from build123d import *

# Parameters (mm, degrees)
BOSS_EXTRUDE1_DEPTH = 3
CUT_EXTRUDE1_DEPTH  = 10


with BuildPart() as part:
    # Sketch2 → Boss-Extrude1 (new body)
    with BuildSketch(Plane.XY):
        with BuildLine():
            Line((-53.128634422, -19.547588701), (-62.746809975, -19.547588701))
            Line((-62.746809975, -19.547588701), (-126.203620945, -19.547588701))
            Line((-126.203620945, -19.547588701), (-126.203620945, 48.452411299))
            ThreePointArc((-126.203620945, 48.452411299), (-118.881290474, 66.130080829), (-101.203620945, 73.452411299))
            Line((-101.203620945, 73.452411299), (-43.703620945, 73.452411299))
            ThreePointArc((-43.703620945, 73.452411299), (-26.025951415, 66.130080829), (-18.703620945, 48.452411299))
            Line((-18.703620945, 48.452411299), (-18.703620945, -51.547588701))
            ThreePointArc((-18.703620945, -51.547588701), (-26.025951415, -69.225258231), (-43.703620945, -76.547588701))
            Line((-43.703620945, -76.547588701), (-101.203620945, -76.547588701))
            ThreePointArc((-101.203620945, -76.547588701), (-118.881290474, -69.225258231), (-126.203620945, -51.547588701))
            Line((-126.203620945, -51.547588701), (-126.203620945, -31.547588701))
            Line((-126.203620945, -31.547588701), (-62.746809975, -31.547588701))
            Line((-62.746809975, -31.547588701), (-53.128634422, -31.547588701))
            ThreePointArc((-53.128634422, -31.547588701), (-47.128634422, -25.547588701), (-53.128634422, -19.547588701))
        make_face()
    extrude(amount=BOSS_EXTRUDE1_DEPTH)

    # Sketch3 → Cut-Extrude1 (cut)
    with BuildSketch(Plane.XY.offset(3)):
        with BuildLine():
            Line((-61.448620945, -37.476562772), (-61.448620945, -68.6318397))
            ThreePointArc((-61.448620945, -68.6318397), (-63.323620945, -70.5068397), (-65.198620945, -68.6318397))
            Line((-65.198620945, -68.6318397), (-65.198620945, -37.476562772))
            ThreePointArc((-65.198620945, -37.476562772), (-63.323620945, -35.601562772), (-61.448620945, -37.476562772))
        make_face()
        with BuildLine():
            Line((-83.458620945, -37.476562772), (-83.458620945, -68.6318397))
            ThreePointArc((-83.458620945, -68.6318397), (-81.583620945, -70.5068397), (-79.708620945, -68.6318397))
            Line((-79.708620945, -68.6318397), (-79.708620945, -37.476562772))
            ThreePointArc((-79.708620945, -37.476562772), (-81.583620945, -35.601562772), (-83.458620945, -37.476562772))
        make_face()
        with BuildLine():
            Line((-83.458620945, -13.61861463), (-83.458620945, 17.536662297))
            ThreePointArc((-83.458620945, 17.536662297), (-81.583620945, 19.411662297), (-79.708620945, 17.536662297))
            Line((-79.708620945, 17.536662297), (-79.708620945, -13.61861463))
            ThreePointArc((-79.708620945, -13.61861463), (-81.583620945, -15.49361463), (-83.458620945, -13.61861463))
        make_face()
        with BuildLine():
            Line((-61.448620945, -13.61861463), (-61.448620945, 17.536662297))
            ThreePointArc((-61.448620945, 17.536662297), (-63.323620945, 19.411662297), (-65.198620945, 17.536662297))
            Line((-65.198620945, 17.536662297), (-65.198620945, -13.61861463))
            ThreePointArc((-65.198620945, -13.61861463), (-63.323620945, -15.49361463), (-61.448620945, -13.61861463))
        make_face()
    extrude(amount=-CUT_EXTRUDE1_DEPTH, mode=Mode.SUBTRACT)


solid = part.part
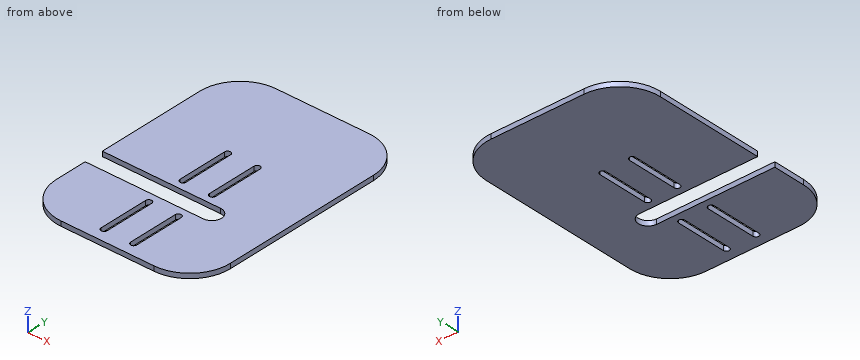
Read the model definition and answer for the solid it produces. Units are mm, in the model's axes. Give positions to 0.01 mm unless a question says otherwise; leave off trailing zeros. Write each loop counter-clockwise with the first axis right and the second up, starting at its lowest first coordinate (ties: lowest second). Pieces come first, ordered by that corner, then holes. Notation, with made-up numbers: (22, -34.75) - (61, -34.75) arc R17 ccw to (61, -16.75) - close; hole circle Ø10 at (16.5, 51). An arc over 180 degrees is marked (long way). Use CSV: the item, a comma, the result in double quotes. Start each with the question number.
(1) Find section D-D (x = -51). Give the vertices of the cut face in (y, z).
(2) Find section B-B (y = 14). Give the vertices of the cut face in (x, z), plus the area to 3 significant figures.
(3) Find section A-A (x = -68.5). Give the vertices of the cut face in (y, z), plus the area to 3 significant figures.
(4) Find section C-C (z = 1.15). Give the vertices of the cut face in (x, y) (3 decimals).
(5) Given P1, Ø1.5, axis at x = -71, y = 18, coming from the -Z side; P2, Ø1.5, axis at y = -60.5, z = 1.5, coming from the -X side, each flat-ended and moving along its own axis, determine where each tip first touches the part or whether it passes through.
(6) Consider line 1 along X through (y, z) = (8, 2.8); line 2 along Y through (x, z) = (-84.5, 1.55); line 3 along X through (y, z) = (-65.5, 0.3). Determine where each line is inside the solid, lowest interval first.
Findings below:
1,outline,"(-76.55, 0) - (-31.16, 0) - (-31.16, 3) - (-76.55, 3) - close; (-19.94, 0) - (73.45, 0) - (73.45, 3) - (-19.94, 3) - close"
2,outline,"(-126.2, 0) - (-83.46, 0) - (-83.46, 3) - (-126.2, 3) - close; (-79.71, 0) - (-65.2, 0) - (-65.2, 3) - (-79.71, 3) - close; (-61.45, 0) - (-18.7, 0) - (-18.7, 3) - (-61.45, 3) - close"
2,area,"300 mm2"
3,outline,"(-76.55, 0) - (-31.55, 0) - (-31.55, 3) - (-76.55, 3) - close; (-19.55, 0) - (73.45, 0) - (73.45, 3) - (-19.55, 3) - close"
3,area,"414 mm2"
4,outline,"(-126.204, -51.548) arc R25 ccw to (-101.204, -76.548) - (-43.704, -76.548) arc R25 ccw to (-18.704, -51.548) - (-18.704, 48.452) arc R25 ccw to (-43.704, 73.452) - (-101.204, 73.452) arc R25 ccw to (-126.204, 48.452) - (-126.204, -19.548) - (-53.129, -19.548) arc R6 cw to (-53.129, -31.548) - (-126.204, -31.548) - close; hole (-83.459, -68.632) arc R1.875 ccw to (-79.709, -68.632) - (-79.709, -37.477) arc R1.875 ccw to (-83.459, -37.477) - close; hole (-83.459, -13.619) arc R1.875 ccw to (-79.709, -13.619) - (-79.709, 17.537) arc R1.875 ccw to (-83.459, 17.537) - close; hole (-65.199, -68.632) arc R1.875 ccw to (-61.449, -68.632) - (-61.449, -37.477) arc R1.875 ccw to (-65.199, -37.477) - close; hole (-65.199, -13.619) arc R1.875 ccw to (-61.449, -13.619) - (-61.449, 17.537) arc R1.875 ccw to (-65.199, 17.537) - close"
5,P1,"z = 0"
5,P2,"x = -124.82"
6,line 1,"-126.2 to -83.46, -79.71 to -65.2, -61.45 to -18.7"
6,line 2,"-76.55 to -31.55, -19.55 to 73.45"
6,line 3,"-121.95 to -83.46, -79.71 to -65.2, -61.45 to -22.96"
